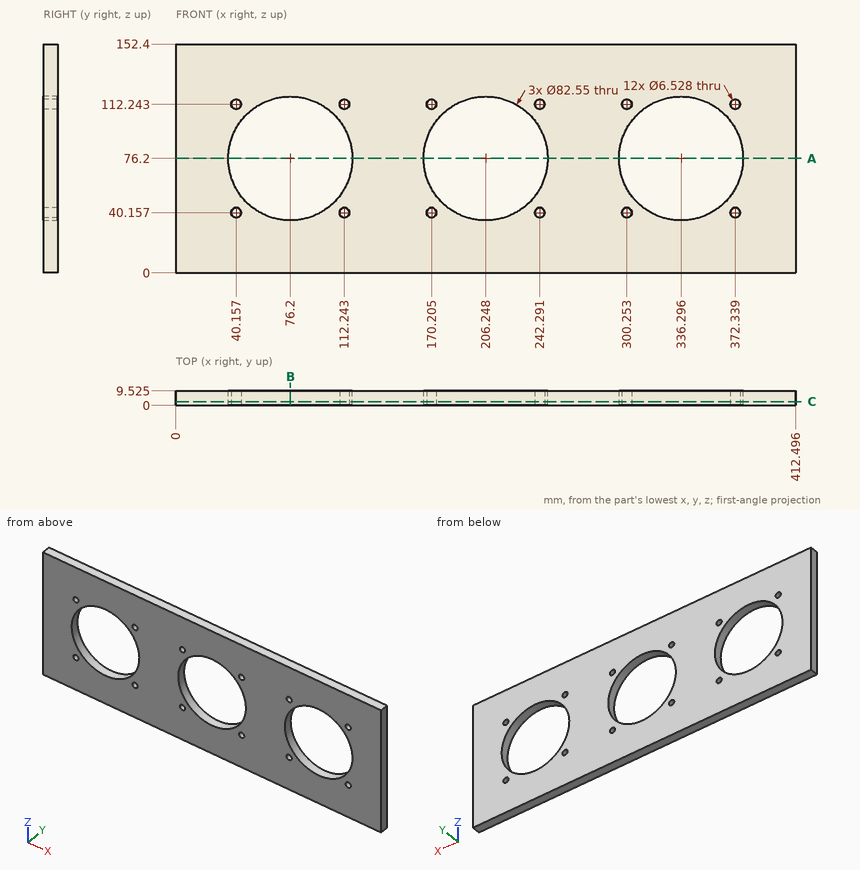
Job drawing, mm, ordinate dimensions from the low corner. One solid piece. Give positions to 0.01 mm unless a question says otherwise; leave off trailing zeros. Loops run counter-clockwise (first coordinate to the right, second up) from the corner with the lowest first, then second, coordinate; pieces in that order, holes last. Notation, with made-up numbers: M 70,-3 L 123,-3 A17 ccw 123,30 Z; hole C 29.25,26 d1. An arc over 180 degrees is marked long. Put each result on its own line as item: value. Start each with the question number.
1) Saw through at A-A (z = 76.2). List the corners of the cut face in (x, y) (1 decimal), then the cut area to 3 significant figures.
2) Probe probe 1 along X at (y, z) = (8.75, 89) (1 decimal); probe 2 along X at (y, z) = (6, 76.2) (1 decimal); probe 3 along Z at (x, y) = (366, 1.25). List the from-to ranges inside material, lowest first.
3) Saw through at C-C (y = 2.5). State how many separate pieces and enclosed holes the cut face has, then the cut area to 3 significant figures.
4) Saw through at B-B (x = 76.2). List the corners of the cut face in (y, z) (1 decimal), then the cut area to 3 significant figures.
Numbers:
1. outline: M 0,0 L 34.9,0 L 34.9,9.5 L 0,9.5 Z; M 117.5,0 L 165,0 L 165,9.5 L 117.5,9.5 Z; M 247.5,0 L 295,0 L 295,9.5 L 247.5,9.5 Z; M 377.6,0 L 412.5,0 L 412.5,9.5 L 377.6,9.5 Z
1. area: 1,570 mm^2
2. probe 1: 0 to 37, 115.4 to 167, 245.5 to 297.1, 375.5 to 412.5
2. probe 2: 0 to 34.9, 117.5 to 165, 247.5 to 295, 377.6 to 412.5
2. probe 3: 0 to 47.54, 104.86 to 152.4
3. separate pieces: 1
3. enclosed holes: 15
3. area: 46,400 mm^2
4. outline: M 0,0 L 9.5,0 L 9.5,34.9 L 0,34.9 Z; M 0,117.5 L 9.5,117.5 L 9.5,152.4 L 0,152.4 Z
4. area: 665 mm^2
